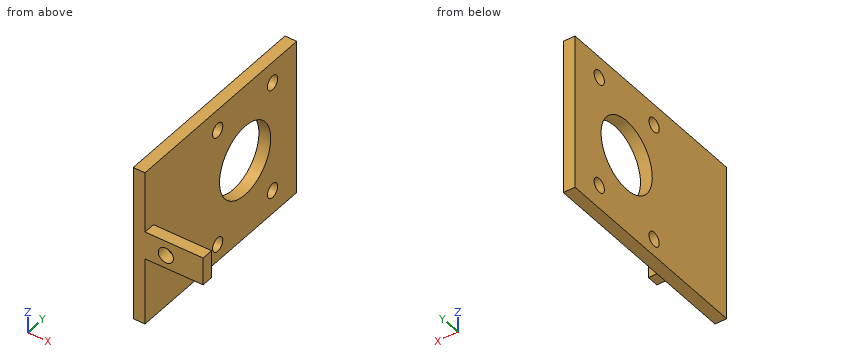
```python
from build123d import *

# Parameters (mm, degrees)
EXTRUDE_THIN2_DEPTH = 30.852042279
SKETCH2_R           = 1.5
CUT_EXTRUDE1_DEPTH  = 53.491563016
SKETCH4_R           = 7
CUT_EXTRUDE3_DEPTH  = 53.491563016
SKETCH6_R           = 1.4
CUT_EXTRUDE5_DEPTH  = 53.491563016
SKETCH7_W           = 16.44057734
SKETCH7_H           = 12.081190297
SKETCH7_H_2         = 13.290689101
CUT_EXTRUDE6_DEPTH  = 53.491563016
SKETCH8_W           = 5.019650722
SKETCH8_H           = 5.480162881
CUT_EXTRUDE7_DEPTH  = 53.491563016


with BuildPart() as part:
    # Sketch1 → Extrude-Thin2 (new body)
    with BuildSketch(Plane.XY):
        Polygon((16.44057734, 0), (0, 0), (0, 39.156392732), (-2.315200758, 39.156392732), (-2.315200758, -2.315200758), (16.44057734, -2.315200758), align=None)
    extrude(amount=-EXTRUDE_THIN2_DEPTH)

    # Sketch2 → Cut-Extrude1 (cut, through all)
    with BuildSketch(Plane(origin=(0, 0, 0), x_dir=(1, 0, 0), z_dir=(0, 1, 0))):
        with Locations(Location((4.097708223, 14.957133601, 0), (0, 0, 270))):
            Circle(SKETCH2_R)
    extrude(amount=-CUT_EXTRUDE1_DEPTH, mode=Mode.SUBTRACT)

    # Sketch4 → Cut-Extrude3 (cut, through all)
    with BuildSketch(Plane(origin=(0, 0, 0), x_dir=(0, 0, -1), z_dir=(1, 0, 0))):
        with Locations((15.188954452, 25.039458811)):
            Circle(SKETCH4_R)
    extrude(amount=-CUT_EXTRUDE3_DEPTH, mode=Mode.SUBTRACT)

    # Sketch6 → Cut-Extrude5 (cut, through all)
    with BuildSketch(Plane(origin=(0, 0, 0), x_dir=(0, 0, -1), z_dir=(1, 0, 0))):
        with Locations((4.188954452, 32.539458811)):
            Circle(SKETCH6_R)
        with Locations((4.188954452, 17.539458811)):
            Circle(SKETCH6_R)
        with Locations((26.188954452, 32.539458811)):
            Circle(SKETCH6_R)
        with Locations((27.46487917, 17.539458811)):
            Circle(SKETCH6_R)
    extrude(amount=-CUT_EXTRUDE5_DEPTH, mode=Mode.SUBTRACT)

    # Sketch7 → Cut-Extrude6 (cut, through all)
    with BuildSketch(Plane(origin=(0, 0, 0), x_dir=(1, 0, 0), z_dir=(0, 1, 0))):
        with Locations((8.22028867, 6.040595149)):
            Rectangle(SKETCH7_W, SKETCH7_H)
        with Locations((8.22028867, 24.206697729)):
            Rectangle(SKETCH7_W, SKETCH7_H_2)
    extrude(amount=-CUT_EXTRUDE6_DEPTH, mode=Mode.SUBTRACT)

    # Sketch8 → Cut-Extrude7 (cut, through all)
    with BuildSketch(Plane(origin=(0, 0, 0), x_dir=(1, 0, 0), z_dir=(0, 1, 0))):
        with Locations((13.930751979, 14.821271738)):
            Rectangle(SKETCH8_W, SKETCH8_H)
    extrude(amount=-CUT_EXTRUDE7_DEPTH, mode=Mode.SUBTRACT)


solid = part.part
```
Source: CAD feature listing. Evaluate the final solid. Frame: model axes, mm. Give positions to 0.01 mm unless a question says otherwise; leave off trailing zeros. Write each loop counter-clockwise with the first axis right and the second up, starting at its lowest first coordinate (ties: lowest second). Pieces come first, ordered by that corner, then holes.
1. Section query C-C (y = 33). Return the cut outline in (x, z), then the cut area to 3 significant figures.
2. Section query B-B (y = 27). Return the cut outline in (x, z), then the cut area to 3 significant figures.
3. First-contact query: pin 1 (2.5 mm diameter, centred on x = 5.5, y = -1.5, fed in from -Z); pin 2 (2.5 mm diameter, centred on y = 17.54, z = -4.19, fed in from +X); pin 3 (1.2 mm diameter, centred on x = 8, y = -1.5, fed in from +Z); pin 4 (3.5 mm diameter, centred on y = 32.54, z = -26.19, fed in from +X). Flat tips, straight axial feed; report the tip coordinate or a pass-through.
4. Section query A-A (z = -25.5). Return the cut outline in (x, y), then the cut area to 3 significant figures.
5. Section query D-D (x = -1.5). Return the cut outline in (y, z).
6. Material intervals for line 1 along X through (y, z) = (10, -11.5); line 2 along Y through (x, z) = (-1, -28.5), sorted ascending.
Output values:
1. outline: (-2.32, -30.85) - (0, -30.85) - (0, -27.51) - (-2.32, -27.51) - close; (-2.32, -24.87) - (0, -24.87) - (0, -5.51) - (-2.32, -5.51) - close; (-2.32, -2.87) - (0, -2.87) - (0, 0) - (-2.32, 0) - close
1. area: 59.2 mm2
2. outline: (-2.32, -30.85) - (0, -30.85) - (0, -21.91) - (-2.32, -21.91) - close; (-2.32, -8.47) - (0, -8.47) - (0, 0) - (-2.32, 0) - close
2. area: 40.3 mm2
3. pin 1: stops at z = -17.56
3. pin 2: passes through
3. pin 3: stops at z = -12.08
3. pin 4: stops at x = 0
4. outline: (-2.32, -2.32) - (0, -2.32) - (0, 31.32) - (-2.32, 31.32) - close; (-2.32, 33.76) - (0, 33.76) - (0, 39.16) - (-2.32, 39.16) - close
4. area: 90.4 mm2
5. outline: (-2.32, -30.85) - (39.16, -30.85) - (39.16, 0) - (-2.32, 0) - close; hole circle Ø2.8 at (17.54, -27.46); hole circle Ø2.8 at (17.54, -4.19); hole circle Ø14 at (25.04, -15.19); hole circle Ø2.8 at (32.54, -26.19); hole circle Ø2.8 at (32.54, -4.19)
6. line 1: x = -2.32 to 0
6. line 2: y = -2.32 to 16.6, 18.48 to 39.16
